Build history of the part. All positions in model axes, mm. Face numbers are marked on the shaded views. Coordinates: 2 decimals unless noted, no trailing zeros. Order: outer loops, then holes, each group sorted by start corner. A loop starts at its lowest first (then second) coordinate and runs counter-clockwise, first axis right, second up. Notation, with made-up numbers: (-16, 88.25) - (22, 88.25) arc R27 ccw to (22, 115.25) - close; hole circle Ø4 at (-20.5, 55.5). An arc over 180 degrees is marked (long way). Return JSON: item names as keys, results as strings.
from build123d import *

# Parameters (mm, degrees)
SKETCH1_R               = 4.765
BOSS_EXTRUDE1_DEPTH     = 9.5
CHAMFER1_SIZE           = 0.76
SKETCH2_R               = 3.43
CUT_EXTRUDE1_DEPTH      = 5.765
CUT_EXTRUDE1_DEPTH_BACK = 5.765


with BuildPart() as part:
    # Sketch1 → Boss-Extrude1 (new body, symmetric)
    with BuildSketch(Plane(origin=(0, 0, 0), x_dir=(0, 0, -1), z_dir=(1, 0, 0))):
        Circle(SKETCH1_R)
    extrude(amount=BOSS_EXTRUDE1_DEPTH, both=True)

    # Chamfer1
    chamfer1_edges = [part.edges().sort_by_distance(p)[0] for p in [
        (-9.5, 0, 4.765),
        (9.5, 0, 4.765),
    ]]
    chamfer(chamfer1_edges, length=CHAMFER1_SIZE)

    # Sketch2 → Cut-Extrude1 (cut, two sides)
    with BuildSketch(Plane(origin=(0, 0, 0), x_dir=(1, 0, 0), z_dir=(0, 1, 0))) as cut_extrude1_sk:
        with Locations((0, -0.25)):
            Circle(SKETCH2_R)
    extrude(amount=CUT_EXTRUDE1_DEPTH, mode=Mode.SUBTRACT)
    extrude(cut_extrude1_sk.sketch, amount=-CUT_EXTRUDE1_DEPTH_BACK, mode=Mode.SUBTRACT)


solid = part.part
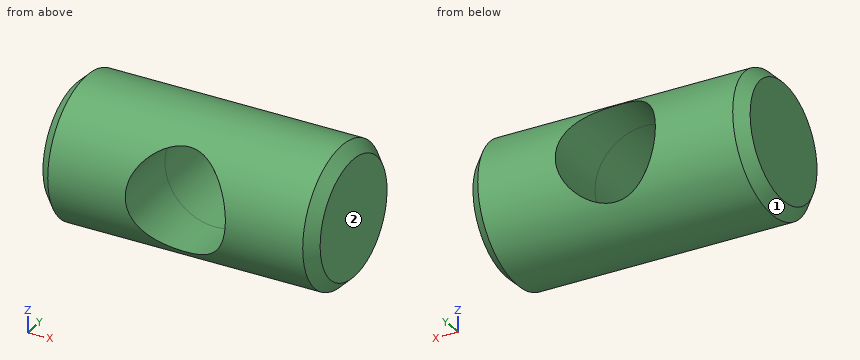
1. Cut at A-A on z = 0. Give the cut face in (x, y) (3 decimals).
Check values:
{"outline": "(-9.5, -4.005) - (-8.74, -4.765) - (-3.421, -4.765) - (-3.421, 4.765) - (-8.74, 4.765) - (-9.5, 4.005) - close; (3.421, -4.765) - (8.74, -4.765) - (9.5, -4.005) - (9.5, 4.005) - (8.74, 4.765) - (3.421, 4.765) - close"}
2. Cut at D-D on x = -2.75. Give the cut face in (y, z) (3 decimals), plus the area to 3 significant figures.
Check values:
{"outline": "(-4.412, -1.8) arc R4.765 ccw to (4.412, -1.8) - close; (-4.173, 2.3) - (4.173, 2.3) arc R4.765 ccw to start", "area": "33.6 mm²"}
3. Probe L1, parallel to X at y = -1.7, z = 0.25; L2, parallel to Z at x = -0.75, y = 0.5; L3, parallel to X at y = -0.75, z = 3. List the from-to ranges inside material, lowest first.
Check values:
{"L1": "-9.5 to -3.43, 3.43 to 9.5", "L2": "-4.74 to -3.1, 3.6 to 4.74", "L3": "-9.5 to -2.05, 2.05 to 9.5"}
4. Cut at B-B on x = 0. Give the cut face in (y, z) (3 decimals), plus the area to 3 significant figures.
Check values:
{"outline": "(-3.549, -3.18) arc R4.765 ccw to (3.549, -3.18) - close; (-3.027, 3.68) - (3.027, 3.68) arc R4.765 ccw to start", "area": "12.3 mm²"}
5. Drop flat-ended pins along their axis: pin 1 (1 mm diameter, centred on x = -4, y = 3.5, fed in from -Z); pin 2 (1 mm diameter, centred on x = -5, z = -1.5, fed in from -Y); pin 3 (4 mm diameter, centred on x = 5.5, y = 1.5, fed in from -Z) (3 decimals); pin 4 (5 mm diameter, centred on x = 5, z = -3.5, fed in from +Y). Give the stop position or say it passes through.
Check values:
{"pin 1": "z = -3.7", "pin 2": "y = -4.66", "pin 3": "z = -4.765", "pin 4": "y = 4.66"}
6. Mould opens along Y. For the marked faces 1 and 2 say: pulls with the +Y half, pulls with the -Y half, needs draft (parallel to the pull), parting line crosses it, or undercut.
Check values:
{"face 1": "parting line crosses it", "face 2": "needs draft"}
7. Cut at C-C on x = 7. Give the cut face in (y, z) (3 decimals).
Check values:
{"outline": "circle Ø9.53 at (0, 0)"}
